Design review of the part built by this model. Coordinates are the model's own, in mm. Face numbers are marked on the shaded views. Give positions to 0.01 mm unless a question says otherwise; leave off trailing zeros. Return JSON: item names as keys, results as strings.
```python
from build123d import *

# Parameters (mm, degrees)
SKETCH2_R           = 2.5
SKETCH2_R_2         = 2
BOSS_EXTRUDE2_DEPTH = 5
CUT_EXTRUDE1_START  = -5
SKETCH3_R           = 2
CUT_EXTRUDE1_DEPTH  = 5


with BuildPart() as part:
    # Sketch1 → Revolve1 (revolve)
    with BuildSketch(Plane.XY, mode=Mode.PRIVATE) as revolve1_sk:
        with BuildLine():
            Line((3.119266055, -4.816513761), (13.119266055, -4.816513761))
            Line((13.119266055, -4.816513761), (13.119266055, -2.816513761))
            Line((13.119266055, -2.816513761), (3.257916771, -2.816513761))
            ThreePointArc((3.257916771, -2.816513761), (-4.025816821, -0.658797724), (-10.372175668, 3.516396035))
            ThreePointArc((-10.372175668, 3.516396035), (-13.131249362, 6.018603225), (-16.672681055, 7.172635302))
            ThreePointArc((-16.672681055, 7.172635302), (-17.771282031, 6.282087215), (-16.880733945, 5.183486239))
            ThreePointArc((-16.880733945, 5.183486239), (-14.048292509, 4.237555299), (-11.880733945, 2.183486239))
            ThreePointArc((-11.880733945, 2.183486239), (-4.911005239, -2.452809391), (3.119266055, -4.816513761))
        make_face()
    revolve(revolve1_sk.sketch.rotate(Axis((13.119266055, -2.816513761, 0), (0, -1, 0)), 270), axis=Axis((13.119266055, -2.816513761, 0), (0, -1, 0)))

    # Sketch2 → Boss-Extrude2 (add)
    # profile 1 of 3: a face of its own
    with BuildSketch(Plane(origin=(0, -2.816513761, 0), x_dir=(1, 0, 0), z_dir=(0, 1, 0))):
        with Locations(Location((9.455762685, 3.402755216, 0), (0, 0, 270))):
            Circle(SKETCH2_R)
        with Locations(Location((9.455762685, 3.402755216, 0), (0, 0, 270))):
            Circle(SKETCH2_R_2, mode=Mode.SUBTRACT)
    # profile 2 of 3: a face of its own
    with BuildSketch(Plane(origin=(0, -2.816513761, 0), x_dir=(1, 0, 0), z_dir=(0, 1, 0))):
        with Locations(Location((17.8978902, 1.471309377, 0), (0, 0, 270))):
            Circle(SKETCH2_R)
        with Locations(Location((17.8978902, 1.471309377, 0), (0, 0, 270))):
            Circle(SKETCH2_R_2, mode=Mode.SUBTRACT)
    # profile 3 of 3: a face of its own
    with BuildSketch(Plane(origin=(0, -2.816513761, 0), x_dir=(1, 0, 0), z_dir=(0, 1, 0))):
        with Locations(Location((12.00414528, -4.874064593, 0), (0, 0, 270))):
            Circle(SKETCH2_R)
        with Locations(Location((12.00414528, -4.874064593, 0), (0, 0, 270))):
            Circle(SKETCH2_R_2, mode=Mode.SUBTRACT)
    extrude(amount=BOSS_EXTRUDE2_DEPTH)

    # Sketch3 → Cut-Extrude1 (cut)
    with BuildSketch(Plane(origin=(0, -2.816513761, 0), x_dir=(1, 0, 0), z_dir=(0, 1, 0)).offset(CUT_EXTRUDE1_START)):
        with Locations(Location((17.8978902, 1.471309377, 0), (0, 0, 90))):
            Circle(SKETCH3_R)
        with Locations(Location((12.00414528, -4.874064593, 0), (0, 0, 90))):
            Circle(SKETCH3_R)
        with Locations(Location((9.455762685, 3.402755216, 0), (0, 0, 90))):
            Circle(SKETCH3_R)
    extrude(amount=CUT_EXTRUDE1_DEPTH, mode=Mode.SUBTRACT)


solid = part.part
```
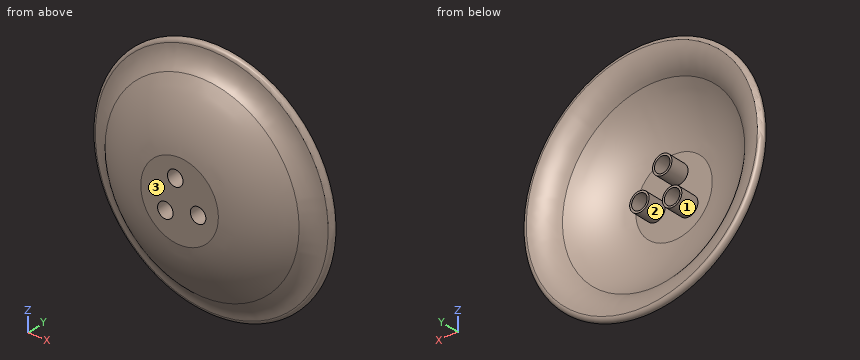
Item 1: For pin 1 (4 mm diameter, centred on x = 36.5, y = 4, fed in from -Z); pin 2 (4.5 mm diameter, centred on x = 12, z = 4.87, fed in from +Y); pin 3 (6 mm diameter, centred on y = -2, z = -5, fed in from +X), all flat-tipped, find the tip position at first contact; note any pin that passes through.
Result set:
{"pin 1": "stops at z = -21.26", "pin 2": "stops at y = 2.18", "pin 3": "stops at x = 36.24"}
Item 2: Add section A-A (y = -2). Give the number of separate pieces and of enclosed holes in the cut face, plus the area to 3 significant figures.
Result set:
{"separate pieces": "4", "enclosed holes": "4", "area": "569 mm^2"}
Item 3: Mouldability with a two-part tool opening along X and no side actions: class the marked faces 1, 2 and 3 as released by +X, released by -X, zero draft, split by the parting line, or undercut.
Result set:
{"face 1": "undercut", "face 2": "undercut", "face 3": "zero draft"}
Item 4: Wall thickness on L1, parallel to Y at x = 8.5, z = 7; L2, parallel to X at y = 1.5, z = 13; L3, parallel to X at y = 0.75, z = -4.5: over which ranges is each line inside the solid? List them lowest first. Write a range as [from, to].
Result set:
{"L1": "y = [-4.82, -2.82]", "L2": "x = [-7.31, -3.28], [29.52, 33.55]", "L3": "x = [-9.73, -6.13], [7.21, 7.78], [11.13, 11.7], [32.37, 35.97]"}
